Input: part model. Units: mm. Frame: model coordinates. Face numbers are marked on the shaded views. Coordinates: 2 decimals unless noted, no trailing zeros. Order: outer loops, then holes, each group sorted by start corner. A loop starts at its lowest first (then second) coordinate and runs counter-clockwise, first axis right, second up. Notation, with made-up numbers: (60.5, 18.25) - (107.5, 18.25) arc R25 cw to (107.5, 30.25) - close; hole circle Ø7 at (1, 88). An arc over 180 degrees is marked (long way). Use a Markdown table: item, result. Add a question column.
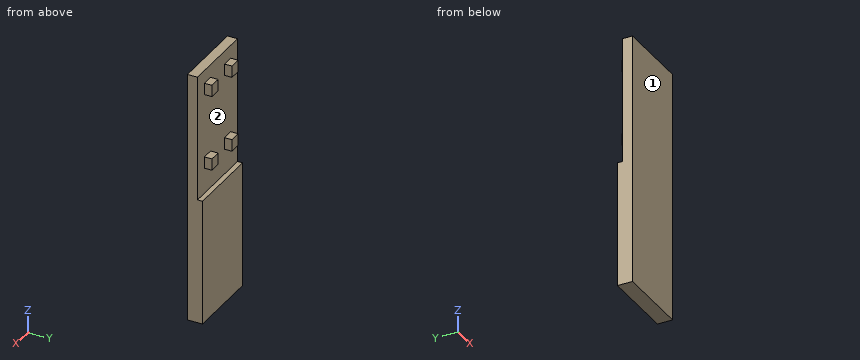
from build123d import *

# Parameters (mm, degrees)
F0_W     = 30
F0_H     = 6
F1_DEPTH = 100
F2_W     = 2
F2_H     = 50
F3_DEPTH = 30
F4_W     = 4.600006
F4_H     = 4.600006
F4_W_2   = 4.600004
F4_H_2   = 4.600004
F4_W_3   = 4.658593
F4_H_3   = 4.717186
F5_DEPTH = 3


with BuildPart() as f1:
    # F0 (on Top) → F1 (new body)
    with BuildSketch(Plane.XY):
        Rectangle(F0_W, F0_H)
    extrude(amount=F1_DEPTH)

    # F2 (on face) → F3 (cut, through all)
    with BuildSketch(Plane.YZ.offset(15)):
        with Locations((2, 75)):
            Rectangle(F2_W, F2_H)
    extrude(amount=-F3_DEPTH, mode=Mode.SUBTRACT)

    # F4 (on face) → F5 (join)
    with BuildSketch(Plane(origin=(0, 1, 0), x_dir=(-1, 0, 0), z_dir=(0, 1, 0))):
        with Locations((-7.5, 92.5)):
            Rectangle(F4_W, F4_H)
        with Locations((7.5, 92.5)):
            Rectangle(F4_W, F4_H)
        with Locations((-7.5, 62.5)):
            Rectangle(F4_W_2, F4_H_2)
        with Locations((7.470703, 62.5)):
            Rectangle(F4_W_3, F4_H_3)
    extrude(amount=F5_DEPTH)


solid = f1.part
1) Material intervals for L1, parallel to Z at x = -9.75, y = 1.5; L2, parallel to Z at x = -6, y = 3.5; L3, parallel to Y at x = 0.75, z = 90, sorted ascending.
2) Contact query for flat-ended pins moving along their axis: P1, Ø0.9, axis at x = -7, y = 3, coming from the -Z side; P2, Ø2.5, axis at y = 3, z = 62, coming from the -X side; P3, Ø3, axis at x = -11, z = 68, coming from the +Y side; P4, Ø2.5, axis at y = 2.5, z = 63, coming from the +X side. Output: stop coordinate, or through.
3) Cut plane A-A (y = 2). Return the cut outline in (x, z).
4) Cut plane B-B (x = -8). Return the cut outline in (y, z).
5) Cut plane D-D (x = 8.5). Return the cut outline in (y, z).
6) Cut plane C-C (z = 93). Return the cut outline in (x, y), and give its area (3 significant figures).
7) Pull-direction query (Z, two-part tool) for the marked faces 1 and 2; classes: pulls with the +Z half, pulls with the -Z half, needs draft (parallel to the pull), parting line crosses it, or undercut.
Computed:
| question | item | result |
|---|---|---|
| 1 | L1 | z = 0 to 50, 60.14 to 64.86, 90.2 to 94.8 |
| 1 | L2 | z = 60.14 to 64.86, 90.2 to 94.8 |
| 1 | L3 | y = -3 to 1 |
| 2 | P1 | stops at z = 0 |
| 2 | P2 | stops at x = -9.8 |
| 2 | P3 | stops at y = 1 |
| 2 | P4 | stops at x = 9.8 |
| 3 | outline | (-15, 0) - (15, 0) - (15, 50) - (-15, 50) - close; (-9.8, 60.14) - (-5.14, 60.14) - (-5.14, 64.86) - (-9.8, 64.86) - close; (-9.8, 90.2) - (-5.2, 90.2) - (-5.2, 94.8) - (-9.8, 94.8) - close; (5.2, 60.2) - (9.8, 60.2) - (9.8, 64.8) - (5.2, 64.8) - close; (5.2, 90.2) - (9.8, 90.2) - (9.8, 94.8) - (5.2, 94.8) - close |
| 4 | outline | (-3, 0) - (3, 0) - (3, 50) - (1, 50) - (1, 60.14) - (4, 60.14) - (4, 64.86) - (1, 64.86) - (1, 90.2) - (4, 90.2) - (4, 94.8) - (1, 94.8) - (1, 100) - (-3, 100) - close |
| 5 | outline | (-3, 0) - (3, 0) - (3, 50) - (1, 50) - (1, 60.2) - (4, 60.2) - (4, 64.8) - (1, 64.8) - (1, 90.2) - (4, 90.2) - (4, 94.8) - (1, 94.8) - (1, 100) - (-3, 100) - close |
| 6 | outline | (-15, -3) - (15, -3) - (15, 1) - (9.8, 1) - (9.8, 4) - (5.2, 4) - (5.2, 1) - (-5.2, 1) - (-5.2, 4) - (-9.8, 4) - (-9.8, 1) - (-15, 1) - close |
| 6 | area | 148 mm2 |
| 7 | face 1 | needs draft |
| 7 | face 2 | undercut |
